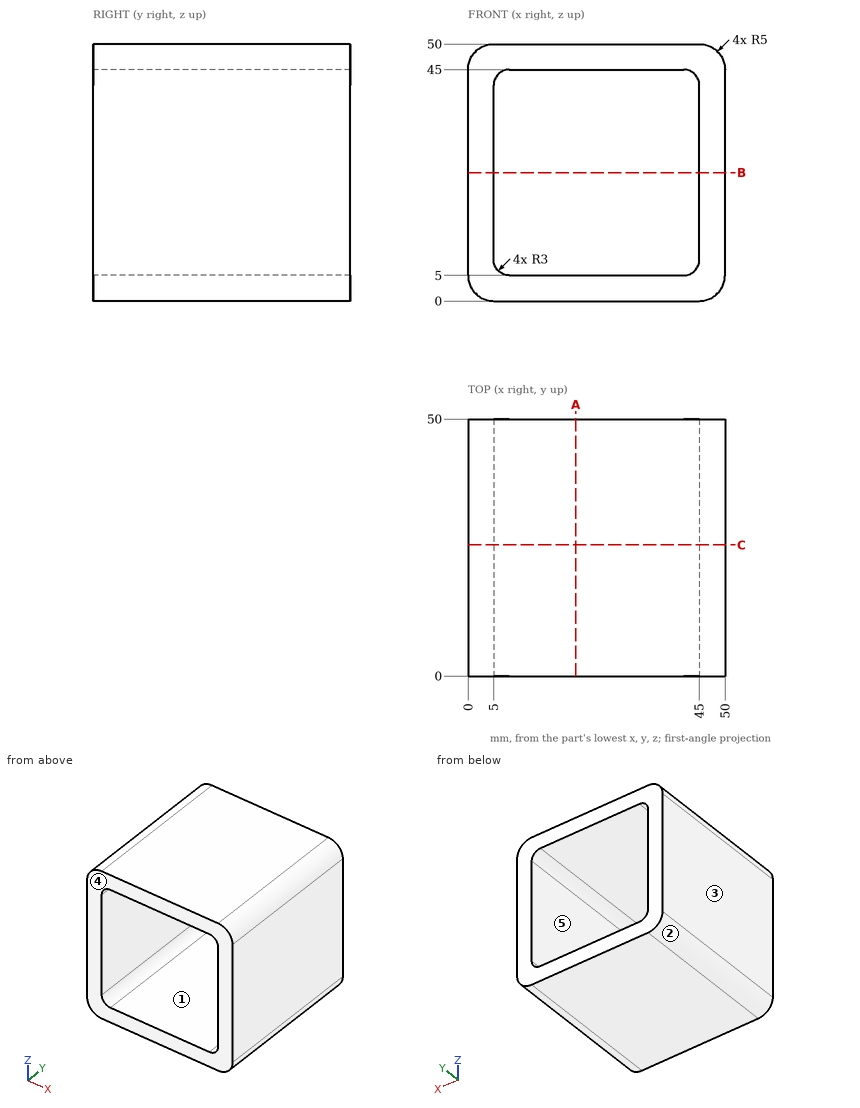
Job drawing, mm, ordinate dimensions from the low corner. One solid piece. A direction names the side the tool comes from. Coordinates: 2 decimals unless noted, no trailing zeros. Order: outer loops, then holes, each group sorted by start corner. A loop starts at its lowest first (then second) coordinate and runs counter-clockwise, first axis right, second up. Notation, with made-up numbers: (-3.5, 42) - (26.5, 42) arc R6 cw to (26.5, 52) - close; hole circle Ø2 at (85.25, 37). An arc over 180 degrees is marked (long way). Return JSON: item names as keys, results as strings. Group by question number.
1) Probe line 1 (Z direction, x = 36, y = 7.5); line 2 (Z direction, x = 6, y = 8.5). List the from-to ranges inside material, lowest first. Write a range as from..to.
2) Saw through at B-B, the plane z = 25. Write the cut outline in (x, y), plus the area to 3 significant figures.
3) Saw through at C-C, the plane y = 25.5. Write the cut outline in (x, z).
4) Saw through at A-A, the plane x = 21. Write the cut outline in (y, z), plus the area to 3 significant figures.
5) Tool access for the marked faces 1 and 2: list every direction of +Z, -Z, +X, -X, +Y, -Y with a clear straight run to the whole face (end or side of a thin tool).
6) Mould opens along X. For the marked faces 3, 4 and 5 say: released by +X, released by -X, zero draft, split by the parting line, or undercut.
Values found:
{
 "1": {"line 1": "z = 0..5, 45..50", "line 2": "z = 0..5.76, 44.24..50"},
 "2": {"outline": "(0, 0) - (5, 0) - (5, 50) - (0, 50) - close; (45, 0) - (50, 0) - (50, 50) - (45, 50) - close", "area": "500 mm²"},
 "3": {"outline": "(0, 5) arc R5 ccw to (5, 0) - (45, 0) arc R5 ccw to (50, 5) - (50, 45) arc R5 ccw to (45, 50) - (5, 50) arc R5 ccw to (0, 45) - close; hole (5, 8) arc R3 ccw to (8, 5) - (42, 5) arc R3 ccw to (45, 8) - (45, 42) arc R3 ccw to (42, 45) - (8, 45) arc R3 ccw to (5, 42) - close"},
 "4": {"outline": "(0, 0) - (50, 0) - (50, 5) - (0, 5) - close; (0, 45) - (50, 45) - (50, 50) - (0, 50) - close", "area": "500 mm²"},
 "5": {"face 1": "+Y, -Y", "face 2": "-Z, -X, +Y, -Y"},
 "6": {"face 3": "released by -X", "face 4": "zero draft", "face 5": "undercut"}
}
